```python
from build123d import *
from OCP.BRepFilletAPI import BRepFilletAPI_MakeChamfer

# Parameters (mm, degrees)
SCHIZZO1_W                   = 100
SCHIZZO1_H                   = 50
ESTRUSIONE_ESTRUSIONE1_DEPTH = 44
SCHIZZO2_W                   = 10.499999851
SCHIZZO2_H                   = 2.500000367
TAGLIO_ESTRUSIONE1_DEPTH     = 106.722514159
TAGLIO_ESTRUSIONE2_DEPTH     = 106.722514247
TAGLIO_ESTRUSIONE3_DEPTH     = 106.722514247
TAGLIO_ESTRUSIONE4_DEPTH     = 106.722514247
SCHIZZO6_W                   = 10.499999851
SCHIZZO6_H                   = 2.500000367
TAGLIO_ESTRUSIONE5_DEPTH     = 106.722514247
SCHIZZO7_W                   = 11.49999996
SCHIZZO7_H                   = 32.999999858
TAGLIO_ESTRUSIONE6_DEPTH     = 106.722514247
TAGLIO_ESTRUSIONE7_REACH     = 115.175
TAGLIO_ESTRUSIONE8_REACH     = 115.175
TAGLIO_ESTRUSIONE9_REACH     = 115.175
TAGLIO_ESTRUSIONE10_REACH    = 115.175
SCHIZZO12_W                  = 14.000000092
SCHIZZO12_H                  = 20
TAGLIO_ESTRUSIONE11_DEPTH    = 106.722514247
FORO_4_0_4_1_D               = 4
FORO_4_0_4_1_DEPTH           = 8.500000443
FORO_4_0_4_2_D               = 4
FORO_4_0_4_2_DEPTH           = 47.500000379
SMUSSO1_SIZE                 = 5
SMUSSO1_SIZE2                = 1
SMUSSO2_SIZE                 = 1.6
SMUSSO3_SIZE                 = 1
SMUSSO3_SIZE2                = 5
RACCORDO1_R                  = 1.5


with BuildPart() as part:
    # Schizzo1 → Estrusione-Estrusione1 (new body)
    with BuildSketch(Plane(origin=(0, 0, -23.5), x_dir=(-1, 0, 0), z_dir=(0, 0, -1))):
        with Locations((-50, 0)):
            Rectangle(SCHIZZO1_W, SCHIZZO1_H)
    extrude(amount=-ESTRUSIONE_ESTRUSIONE1_DEPTH)

    # Schizzo2 → Taglio-Estrusione1 (cut, through all)
    with BuildSketch(Plane.ZY):
        with Locations((15.250000075, -23.750000189)):
            Rectangle(SCHIZZO2_W, SCHIZZO2_H)
    extrude(amount=-TAGLIO_ESTRUSIONE1_DEPTH, mode=Mode.SUBTRACT)

    # Schizzo3 → Taglio-Estrusione2 (cut, through all)
    with BuildSketch(Plane.ZY):
        Polygon((-2.5, -25), (2.5, -25), (2.5, -22.5), (7, -22.5), (7, -12.5), (-7, -12.5), (-7, -22.5), (-2.5, -22.5), align=None)
    extrude(amount=-TAGLIO_ESTRUSIONE2_DEPTH, mode=Mode.SUBTRACT)

    # Schizzo4 → Taglio-Estrusione3 (cut, through all)
    with BuildSketch(Plane.ZY):
        Polygon((-23.5, 9.5), (-23.5, -9.5), (-20.5, -9.5), (-20.5, -22.5), (-9, -22.5), (-9, 22.5), (-20.5, 22.5), (-20.5, 9.5), align=None)
    extrude(amount=-TAGLIO_ESTRUSIONE3_DEPTH, mode=Mode.SUBTRACT)

    # Schizzo5 → Taglio-Estrusione4 (cut, through all)
    with BuildSketch(Plane.ZY):
        Polygon((2.5, 25), (-2.5, 25), (-2.5, 22.5), (-7, 22.5), (-7, 12.5), (7, 12.5), (7, 22.5), (2.5, 22.5), align=None)
    extrude(amount=-TAGLIO_ESTRUSIONE4_DEPTH, mode=Mode.SUBTRACT)

    # Schizzo6 → Taglio-Estrusione5 (cut, through all)
    with BuildSketch(Plane.ZY):
        with Locations((15.250000075, 23.750000189)):
            Rectangle(SCHIZZO6_W, SCHIZZO6_H)
    extrude(amount=-TAGLIO_ESTRUSIONE5_DEPTH, mode=Mode.SUBTRACT)

    # Schizzo7 → Taglio-Estrusione6 (cut, through all)
    with BuildSketch(Plane.ZY):
        with Locations((14.75000002, 0)):
            Rectangle(SCHIZZO7_W, SCHIZZO7_H)
    extrude(amount=-TAGLIO_ESTRUSIONE6_DEPTH, mode=Mode.SUBTRACT)

    # Schizzo8 → Taglio-Estrusione7 (cut, up to next)
    with BuildSketch(Plane(origin=(0, 22.500000006, 0), x_dir=(-1, 0, 0), z_dir=(0, 1, 0)), mode=Mode.PRIVATE) as taglio_estrusione7_sk1:
        with BuildLine():
            Line((-75, 11.500000046), (-55, 11.500000046))
            ThreePointArc((-55, 11.500000046), (-52, 14.500000046), (-55, 17.500000046))
            Line((-55, 17.500000046), (-75, 17.500000046))
            ThreePointArc((-75, 17.500000046), (-78, 14.500000046), (-75, 11.500000046))
        make_face()
    taglio_estrusione7_tool1 = extrude(taglio_estrusione7_sk1.sketch, amount=-TAGLIO_ESTRUSIONE7_REACH, mode=Mode.PRIVATE) & part.part
    add(taglio_estrusione7_tool1.solids().sort_by_distance((65, 22.5, 14.5))[0], mode=Mode.SUBTRACT)

    # Schizzo9 → Taglio-Estrusione8 (cut, up to next)
    with BuildSketch(Plane(origin=(0, 22.500000006, 0), x_dir=(-1, 0, 0), z_dir=(0, 1, 0)), mode=Mode.PRIVATE) as taglio_estrusione8_sk1:
        with BuildLine():
            Line((-25, 17.500000046), (-45, 17.500000046))
            ThreePointArc((-45, 17.500000046), (-48, 14.500000046), (-45, 11.500000046))
            Line((-45, 11.500000046), (-25, 11.500000046))
            ThreePointArc((-25, 11.500000046), (-22, 14.500000046), (-25, 17.500000046))
        make_face()
    taglio_estrusione8_tool1 = extrude(taglio_estrusione8_sk1.sketch, amount=-TAGLIO_ESTRUSIONE8_REACH, mode=Mode.PRIVATE) & part.part
    add(taglio_estrusione8_tool1.solids().sort_by_distance((35, 22.5, 14.5))[0], mode=Mode.SUBTRACT)

    # Schizzo10 → Taglio-Estrusione9 (cut, up to next)
    with BuildSketch(Plane.XZ.offset(22.500000006), mode=Mode.PRIVATE) as taglio_estrusione9_sk1:
        with BuildLine():
            Line((55, 11.500000046), (75, 11.500000046))
            ThreePointArc((75, 11.500000046), (78, 14.500000046), (75, 17.500000046))
            Line((75, 17.500000046), (55, 17.500000046))
            ThreePointArc((55, 17.500000046), (52, 14.500000046), (55, 11.500000046))
        make_face()
    taglio_estrusione9_tool1 = extrude(taglio_estrusione9_sk1.sketch, amount=-TAGLIO_ESTRUSIONE9_REACH, mode=Mode.PRIVATE) & part.part
    add(taglio_estrusione9_tool1.solids().sort_by_distance((65, -22.5, 14.5))[0], mode=Mode.SUBTRACT)

    # Schizzo11 → Taglio-Estrusione10 (cut, up to next)
    with BuildSketch(Plane.XZ.offset(22.500000006), mode=Mode.PRIVATE) as taglio_estrusione10_sk1:
        with BuildLine():
            Line((45, 17.500000046), (25, 17.500000046))
            ThreePointArc((25, 17.500000046), (22, 14.500000046), (25, 11.500000046))
            Line((25, 11.500000046), (45, 11.500000046))
            ThreePointArc((45, 11.500000046), (48, 14.500000046), (45, 17.500000046))
        make_face()
    taglio_estrusione10_tool1 = extrude(taglio_estrusione10_sk1.sketch, amount=-TAGLIO_ESTRUSIONE10_REACH, mode=Mode.PRIVATE) & part.part
    add(taglio_estrusione10_tool1.solids().sort_by_distance((35, -22.5, 14.5))[0], mode=Mode.SUBTRACT)

    # Schizzo12 → Taglio-Estrusione11 (cut, through all)
    with BuildSketch(Plane.ZY):
        Rectangle(SCHIZZO12_W, SCHIZZO12_H)
    extrude(amount=-TAGLIO_ESTRUSIONE11_DEPTH, mode=Mode.SUBTRACT)

    # Foro Ø4.0 (4)-1
    with Locations(Plane(origin=(0, 16.499999929, 0), x_dir=(-1, 0, 0), z_dir=(0, -1, 0))):
        with Locations((-85, -14.500000203), (-15, -14.500000203)):
            Hole(FORO_4_0_4_1_D / 2, depth=FORO_4_0_4_1_DEPTH)

    # Foro Ø4.0 (4)-2
    with Locations(Plane(origin=(0, -22.500000006, 0), x_dir=(-1, 0, 0), z_dir=(0, -1, 0))):
        with Locations((-85, -14.5), (-15, -14.5)):
            Hole(FORO_4_0_4_2_D / 2, depth=FORO_4_0_4_2_DEPTH)

    # Smusso1: one chamfer whose edges measure the first distance from different faces: ONE call of the kernel's chamfer builder (chamfer() names one face for all edges)
    smusso1_edges_1 = [part.edges().sort_by_distance(p)[0] for p in [
        (100, 16.499999929, 14.75000002),
    ]]
    smusso1_side_1 = [part.faces().sort_by_distance(p)[0] for p in [
        (50, 16.499999929, 14.847088678),
    ]]
    smusso1_edges_2 = [part.edges().sort_by_distance(p)[0] for p in [
        (0, -16.499999929, 14.75000002),
    ]]
    smusso1_side_2 = [part.faces().sort_by_distance(p)[0] for p in [
        (0, -17.25, -22.833966968),
    ]]
    smusso1 = BRepFilletAPI_MakeChamfer(part.part.solid().wrapped)
    for e in smusso1_edges_1:
        smusso1.Add(SMUSSO1_SIZE, SMUSSO1_SIZE2, e.wrapped, smusso1_side_1[0].wrapped)  # the first distance lies on this face
    for e in smusso1_edges_2:
        smusso1.Add(SMUSSO1_SIZE, SMUSSO1_SIZE2, e.wrapped, smusso1_side_2[0].wrapped)  # the first distance lies on this face
    add(Compound.cast(smusso1.Shape()), mode=Mode.REPLACE)

    # Smusso2
    smusso2_edges = [part.edges().sort_by_distance(p)[0] for p in [
        (50, 12.5, 7),
        (50, 12.5, -7),
        (50, 22.5, -7),
        (50, -22.5, -7),
        (50, -12.5, -7),
        (50, -12.5, 7),
        (50, -22.5, 7),
        (50, 22.5, 7),
    ]]
    chamfer(smusso2_edges, length=SMUSSO2_SIZE)

    # Smusso3: one chamfer whose edges measure the first distance from different faces: ONE call of the kernel's chamfer builder (chamfer() names one face for all edges)
    smusso3_edges_1 = [part.edges().sort_by_distance(p)[0] for p in [
        (100, -16.499999929, 14.75000002),
    ]]
    smusso3_side_1 = [part.faces().sort_by_distance(p)[0] for p in [
        (100, -23.166033032, 3.95),
    ]]
    smusso3_edges_2 = [part.edges().sort_by_distance(p)[0] for p in [
        (0, 16.499999929, 14.75000002),
    ]]
    smusso3_side_2 = [part.faces().sort_by_distance(p)[0] for p in [
        (47.5, 16.499999929, 19.543064788),
    ]]
    smusso3 = BRepFilletAPI_MakeChamfer(part.part.solid().wrapped)
    for e in smusso3_edges_1:
        smusso3.Add(SMUSSO3_SIZE, SMUSSO3_SIZE2, e.wrapped, smusso3_side_1[0].wrapped)  # the first distance lies on this face
    for e in smusso3_edges_2:
        smusso3.Add(SMUSSO3_SIZE, SMUSSO3_SIZE2, e.wrapped, smusso3_side_2[0].wrapped)  # the first distance lies on this face
    add(Compound.cast(smusso3.Shape()), mode=Mode.REPLACE)

    # Raccordo1
    raccordo1_edges = [part.edges().sort_by_distance(p)[0] for p in [
        (50, -10, 7.000000046),
        (50, -10, -7.000000046),
        (50, 10, -7.000000046),
        (50, 10, 7.000000046),
        (50, 22.5, -20.5),
        (50, 22.5, -9),
        (50, -22.5, -9),
        (50, -22.5, -20.5),
    ]]
    fillet(raccordo1_edges, radius=RACCORDO1_R)


solid = part.part
```
For this review, take the finished solid that the model builds, in its own axes (mm). A direction names the side the tool comes from. Round coordinates to 2 decimals unless told otherwise and drop trailing zeros. Write each loop counter-clockwise with the first axis right and the second up, starting at its lowest first coordinate (ties: lowest second). Pieces come first, ordered by that corner, then holes. Notation, with made-up numbers: M 60,-37.5 L 109,-37.5 A9 ccw 109,-27.5 Z; hole C 54.5,76 d9. An arc over 180 degrees is marked long. One line per item, written item: value. Start each with the question number.
(1) Insertion check: pin 1 (6 mm diameter, centred on y = 2, z = 4.5, fed in from -X); pin 2 (1.2 mm diameter, centred on x = 49.5, y = 24, fed in from +Z); pin 3 (6 mm diameter, centred on x = 82, y = 8, fed in from +Z); pin 4 (8.5 mm diameter, centred on x = 30, z = 17, fed in from +Y). Each pin has a flat end and moves straight along its axis. Give the tip position at first contact, or say it passes through.
(2) We need section A-A (y = -4). Give the boundary of the cut face in (x, z), and give its area (3 significant figures).
(3) We need section B-B (x = 85). Count the separate pieces of the cut face and the enclosed holes in it, and give its area (3 significant figures).
(4) Wall thickness on line 1 (Z direction, x = 42.5, y = -20.5); line 2 (Z direction, x = 15, y = -20); line 3 (Z direction, x = 21, y = 10.5): over which ranges is each line inside the solid? List them lowest first.
(5) The part is to be moulded in two halves that separate along Y. For faces 5 (the flat face through (35, 20, 17.5)), 6 (the flat face through (49, -22.5, 15)), 7 (the flat face through (0.5, 19, 14.7)), say which applies: released by +Y, released by -Y, zero draft, split by the parting line, or undercut.
(6) Machinability: for faces 1 (the flat face through (47, -16.5, 12)), 2 (the flat face through (49, 17, 7)), 3 (the cylindrical face through (52, 19.5, 14.4)), 4 (the flat face through (49, 24, -2.5)), which of the approach directions +Z, -Z, +X, -X, +Y, -Y give a long, thin tool a straight path to every point of the face, cutting with its end or side? Answer none if there is none.
Result:
1. pin 1: x = 0
1. pin 2: z = 10
1. pin 3: z = 9
1. pin 4: y = 22.5
2. outline: M 0,-9 L 100,-9 L 100,-7 L 0,-7 Z; M 0,7 L 100,7 L 100,9 L 0,9 Z
2. area: 400 mm²
3. separate pieces: 3
3. enclosed holes: 1
3. area: 575 mm²
4. line 1: -23.5 to -20.5, -9 to -7, 7 to 11.5, 17.5 to 20.5
4. line 2: -23.5 to -20.5, -9 to -7, 7 to 12.5, 16.5 to 20.5
4. line 3: -23.5 to -20.5, -9 to 9
5. face 5: zero draft
5. face 6: released by -Y
5. face 7: undercut
6. face 1: +Z, +X, -X
6. face 2: +X, -X
6. face 3: +Y, -Y
6. face 4: +X, -X, +Y
